Input: part model. Units: mm. Frame: model coordinates. Face numbers are marked on the shaded views. A direction names the side the tool comes from. Coordinates: 2 decimals unless noted, no trailing zeros. Write each loop counter-clockwise with the first axis right and the second up, starting at its lowest first coordinate (ties: lowest second). Pieces come first, ordered by that corner, then holes. Notation, with made-up numbers: M -1,83.5 L 13,83.5 A12 ccw 13,90.5 Z; hole C -7,48 d1. An arc over 180 degrees is marked long. Write each question's results on one line, items separated by ' | '. Start each with the question number.
1. Ray query, probe 1 along Y at (x, z) = (0, 1); probe 2 along X at (y, z) = (1.5, 23); probe 3 along Y at (x, z) = (-43, 9.5). Return the intervals inside material, ascending.
2. Section query D-D, the plane y = -1.5. Output: boundary loops of the cut face in (x, z).
3. Set-up query: the marked faces 1 and 2. Return all of +Z, -Z, +X, -X, +Y, -Y with unobstructed straight access to the full face (end or side cutting, diameter ignored); none if empty.
4. Section query C-C, the plane y = -53. Output: boundary loops of the cut face in (x, z), and give its area (3 significant figures).
5. Section query A-A, the plane z = 36. Output: boundary loops of the cut face in (x, y), and give its area (3 significant figures).
6. First-contact query: pin 1 (1 mm diameter, centred on x = 3.5, z = 12, fed in from -Y); pin 2 (4 mm diameter, centred on x = -11, y = -47.5, fed in from +Z). Flat tips, straight axial feed; report the tip coordinate or a pass-through.
7. Section query B-B, the plane x = 0. Output: boundary loops of the cut face in (y, z), and give its area (3 significant figures).
8. Pull-direction query (X, two-part tool) for the marked faces 3, 4 and 5; classes: +X half, -X half, draft (parallel to the pull), parting line (faces both ways), or undercut.
```python
from build123d import *

# Parameters (mm, degrees)
F0_W     = 119.634
F0_H     = 178.054
F1_DEPTH = 68.58
F2_W     = 114.554
F2_H     = 172.974
F3_DEPTH = 64.77
F5_DEPTH = 190.5
F6_R     = 12.7
F7_DEPTH = 5.08


with BuildPart() as f1:
    # F0 (on Top) → F1 (new body)
    with BuildSketch(Plane.XY):
        Rectangle(F0_W, F0_H)
    extrude(amount=F1_DEPTH)

    # F2 (on face) → F3 (cut)
    with BuildSketch(Plane.XY.offset(68.58)):
        Rectangle(F2_W, F2_H)
    extrude(amount=-F3_DEPTH, mode=Mode.SUBTRACT)

    # F4 (on face) → F5 (cut)
    with BuildSketch(Plane.XZ.offset(89.027)):
        with BuildLine():
            ThreePointArc((-12.7, 21.965362), (0, 9.265362), (12.7, 21.965362))
            ThreePointArc((12.7, 21.965362), (0, 34.665362), (-12.7, 21.965362))
        make_face()
        with BuildLine():
            ThreePointArc((-12.7, 21.965362), (0, 34.665362), (12.7, 21.965362))
            Line((12.7, 21.965362), (12.7, 68.58))
            Line((12.7, 68.58), (-12.7, 68.58))
            Line((-12.7, 68.58), (-12.7, 21.965362))
        make_face()
    extrude(amount=-F5_DEPTH, mode=Mode.SUBTRACT)

    # F6 (on face) → F7 (cut)
    with BuildSketch(Plane(origin=(0, 0, 0), x_dir=(1, 0, 0), z_dir=(0, 0, -1))):
        with Locations((0, 57.277)):
            Circle(F6_R)
        with Locations((0, -57.277)):
            Circle(F6_R)
    extrude(amount=-F7_DEPTH, mode=Mode.SUBTRACT)


solid = f1.part
```
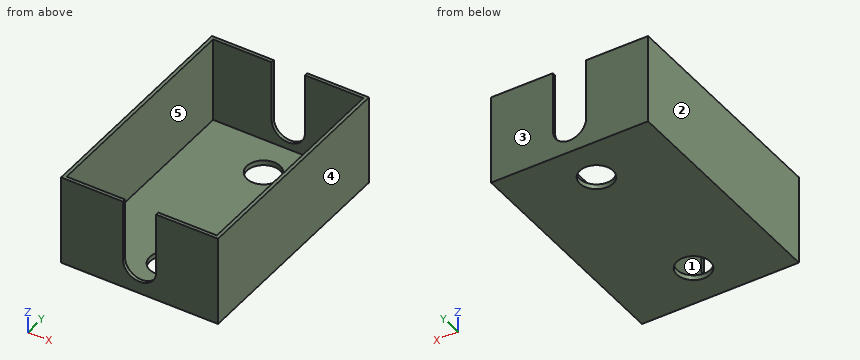
Answer:
1) probe 1: -89.03 to -69.98, -44.58 to 44.58, 69.98 to 89.03 | probe 2: -59.82 to -57.28, 57.28 to 59.82 | probe 3: -89.03 to -86.49, 86.49 to 89.03
2) outline: M -59.82,0 L 59.82,0 L 59.82,68.58 L 57.28,68.58 L 57.28,3.81 L -57.28,3.81 L -57.28,68.58 L -59.82,68.58 Z
3) face 1: +Z | face 2: +Z, -Z, -X, +Y, -Y
4) outline: M -59.82,0 L -11.96,0 L -11.96,3.81 L -57.28,3.81 L -57.28,68.58 L -59.82,68.58 Z; M 11.96,0 L 59.82,0 L 59.82,68.58 L 57.28,68.58 L 57.28,3.81 L 11.96,3.81 Z | area: 694 mm^2
5) outline: M -59.82,-89.03 L -12.7,-89.03 L -12.7,-86.49 L -57.28,-86.49 L -57.28,86.49 L -12.7,86.49 L -12.7,89.03 L -59.82,89.03 Z; M 12.7,-89.03 L 59.82,-89.03 L 59.82,89.03 L 12.7,89.03 L 12.7,86.49 L 57.28,86.49 L 57.28,-86.49 L 12.7,-86.49 Z | area: 1,360 mm^2
6) pin 1: through | pin 2: z = 3.81
7) outline: M -89.03,0 L -69.98,0 L -69.98,3.81 L -86.49,3.81 L -86.49,9.27 L -89.03,9.27 Z; M -44.58,0 L 44.58,0 L 44.58,3.81 L -44.58,3.81 Z; M 69.98,0 L 89.03,0 L 89.03,9.27 L 86.49,9.27 L 86.49,3.81 L 69.98,3.81 Z | area: 513 mm^2
8) face 3: draft | face 4: +X half | face 5: undercut
